Source: three-view drawing plus pictorial views. Frame: mm from the lowest corner of the part. A direction names the side the tool comes from. Give positions to 0.01 mm unless a question says otherwise; leave off trailing zeros. Order: outer loops, then holes, each group sorted by start corner. A loop starts at its lowest first (then second) coordinate and runs counter-clockwise, first axis right, second up. Notation, with made-up numbers: M 43,78 L 47,78 A20 cw 47,115 Z; hole C -16.75,74.5 d5. An arc over 180 degrees is marked long. Use CSV: the item, a comma, the result in double quotes. Start each with the question number.
Item 1: Section query B-B on y = 6. Return loops of the section in (x, z).
Item 2: Ray query, probe 1 along Z at (x, y) = (45, 6.15); probe 2 along X at (y, z) = (8.95, 29.25); probe 3 along X at (y, z) = (4.5, 37.5). Return the intervals inside material, ascending. Write a range as from..to.
Item 3: Access query for the marked faces 1 and 2. Directions: +Z, -Z, +X, -X, +Y, -Y. A direction counts if a zero-diameter tool reaches every point of the face in a straight line with its end or side. Return the directions, or none.
Item 4: Section query D-D on y = 1. Return loops of the section in (x, z).
Item 5: Section query A-A on z = 39. Return loops of the section in (x, y), and give its area (3 significant figures).
Item 6: Section query C-C on x = 18. Return loops of the section in (y, z), and give its area (3 significant figures).
Item 7: Pull-direction query (X, two-part tool) for the marked faces 3 and 4; classes: +X half, -X half, draft (parallel to the pull), parting line (faces both ways), or undercut.
Item 8: First-contact query: pin 1 (4.5 mm diameter, centred on x = 63, z = 16.25, fed in from +Y); pin 2 (1.5 mm diameter, centred on y = 9, z = 31, fed in from +X); pin 3 (4 mm diameter, centred on x = 18.5, z = 48, fed in from -Y). Flat tips, straight axial feed; report the tip coordinate or a pass-through.
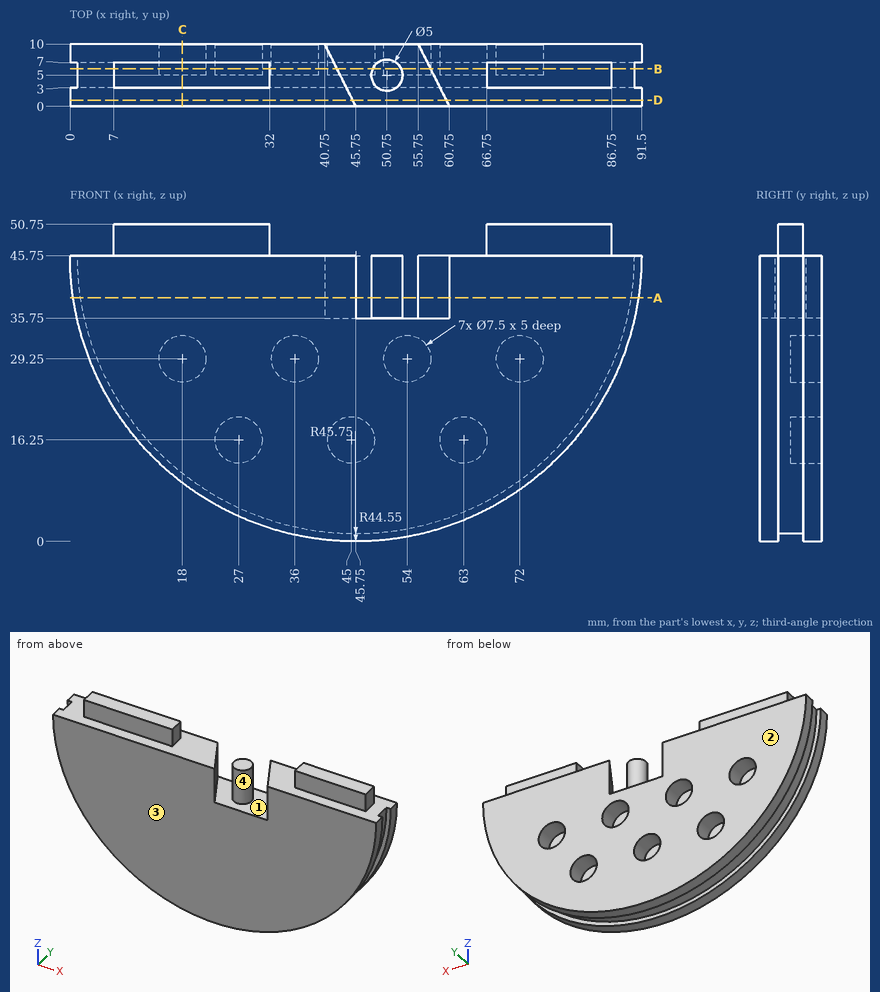
Verdict:
1,outline,"M 1.2,45.75 A44.55 ccw 90.3,45.75 L 86.75,45.75 L 86.75,50.75 L 66.75,50.75 L 66.75,45.75 L 57.75,45.75 L 57.75,35.75 L 53.04,35.75 L 53.04,45.75 L 48.46,45.75 L 48.46,35.75 L 42.75,35.75 L 42.75,45.75 L 32,45.75 L 32,50.75 L 7,50.75 L 7,45.75 Z; hole C 18,29.25 d7.5; hole C 27,16.25 d7.5; hole C 36,29.25 d7.5; hole C 45,16.25 d7.5; hole C 54,29.25 d7.5; hole C 63,16.25 d7.5; hole C 72,29.25 d7.5"
2,probe 1,"1.21..12.5, 20..35.75"
2,probe 2,"3.08..14.25, 21.75..32.25, 39.75..50.25, 57.75..68.25, 75.75..88.42"
2,probe 3,"1.97..43.5, 48.3..53.2, 58.5..89.53"
3,face 1,"+Z"
3,face 2,"+Z, -Z, +X, -X, +Y"
4,outline,"M 0,45.75 A45.75 ccw 91.5,45.75 L 60.25,45.75 L 60.25,35.75 L 45.25,35.75 L 45.25,45.75 Z"
5,outline,"M 0.5,0 L 45.75,0 L 40.75,10 L 0.5,10 L 0.5,7 L 1.71,7 L 1.71,3 L 0.5,3 Z; C 50.75,5 d5; M 55.75,10 L 60.75,0 L 91,0 L 91,3 L 89.79,3 L 89.79,7 L 91,7 L 91,10 Z"
5,area,"765 mm2"
6,outline,"M 0,9.38 L 3,9.38 L 3,10.9 L 7,10.9 L 7,9.38 L 10,9.38 L 10,25.5 L 5,25.5 L 5,33 L 10,33 L 10,45.75 L 7,45.75 L 7,50.75 L 3,50.75 L 3,45.75 L 0,45.75 Z"
6,area,"340 mm2"
7,face 3,"draft"
7,face 4,"undercut"
8,pin 1,"y = 5"
8,pin 2,"x = 89.31"
8,pin 3,"y = 3"
